from build123d import *

# Parameters (mm, degrees)
BOSS_EXTRUDE4_DEPTH  = 1.5875
M3_CLEARANCE_HOLE3_D = 3
M3_CLEARANCE_HOLE1_D = 3.1
M3_CLEARANCE_HOLE4_D = 2.95
M3_CLEARANCE_HOLE2_D = 3.1
BOSS_EXTRUDE6_DEPTH  = 3.175
FILLET1_R            = 2
FILLET3_R            = 1
FILLET6_R            = 0.5
CUT_EXTRUDE4_DEPTH   = 10
SKETCH29_R           = 1.5
CUT_EXTRUDE5_DEPTH   = 10
SKETCH31_R           = 1.5
CUT_EXTRUDE7_DEPTH   = 10


with BuildPart() as part:
    # Sketch1 → Boss-Extrude4 (new, symmetric)
    with BuildSketch(Plane(origin=(0, 0, 0), x_dir=(1, 0, 0), z_dir=(0, 1, 0))):
        with BuildLine():
            Line((-62.799553621, 32.496136604), (-73.969425011, 32.691107434))
            Line((-73.969425011, 32.691107434), (-77.053684287, 35.88495141))
            ThreePointArc((-77.053684287, 35.88495141), (-84.36642289, 10.358894189), (-83.446216027, -16.178041625))
            Line((-83.446216027, -16.178041625), (-79.680911643, -13.825218315))
            Line((-79.680911643, -13.825218315), (-69.484649137, -16.179210996))
            Line((-69.484649137, -16.179210996), (-43.894490772, -57.132025032))
            Line((-43.894490772, -57.132025032), (-43.894490772, -64.826600275))
            Line((-43.894490772, -64.826600275), (-43.094490772, -64.826600275))
            Line((-43.094490772, -64.826600275), (-34, -64.826600275))
            Line((-34, -64.826600275), (-34, -59.55))
            Line((-34, -59.55), (-34, -58.55))
            Line((-34, -58.55), (-20, -58.55))
            Line((-20, -58.55), (-19.859459165, -59.55))
            Line((-19.859459165, -59.55), (19.859459165, -59.55))
            Line((19.859459165, -59.55), (20, -58.55))
            Line((20, -58.55), (34, -58.55))
            Line((34, -58.55), (34, -59.55))
            Line((34, -59.55), (34, -64.826600275))
            Line((34, -64.826600275), (43.094490772, -64.826600275))
            Line((43.094490772, -64.826600275), (43.894490772, -64.826600275))
            Line((43.894490772, -64.826600275), (43.894490772, -57.132025032))
            Line((43.894490772, -57.132025032), (69.484649137, -16.179210996))
            Line((69.484649137, -16.179210996), (79.680911643, -13.825218315))
            Line((79.680911643, -13.825218315), (83.446216027, -16.178041625))
            ThreePointArc((83.446216027, -16.178041625), (84.610662337, -8.126242604), (85, 0))
            ThreePointArc((85, 0), (82.98964744, 18.377116688), (77.053684287, 35.88495141))
            Line((77.053684287, 35.88495141), (73.969425011, 32.691107434))
            Line((73.969425011, 32.691107434), (62.799553621, 32.496136604))
            Line((62.799553621, 32.496136604), (30.284668021, 63.895396642))
            Line((30.284668021, 63.895396642), (30.089697191, 75.065268032))
            Line((30.089697191, 75.065268032), (33.173956467, 78.259112008))
            ThreePointArc((33.173956467, 78.259112008), (0, 85), (-33.173956467, 78.259112008))
            Line((-33.173956467, 78.259112008), (-30.089697191, 75.065268032))
            Line((-30.089697191, 75.065268032), (-30.284668021, 63.895396642))
            Line((-30.284668021, 63.895396642), (-62.799553621, 32.496136604))
        make_face()
    extrude(amount=BOSS_EXTRUDE4_DEPTH, both=True)

    # M3 Clearance Hole3 (through all)
    with Locations(Plane(origin=(0, -1.5875, 0), x_dir=(-1, 0, 0), z_dir=(0, -1, 0))):
        with Locations((36.5, -50), (36.5, -38), (-36.5, -50), (-36.5, -38)):
            Hole(M3_CLEARANCE_HOLE3_D / 2)

    # M3 Clearance Hole1 (through all)
    with Locations(Plane(origin=(0, 1.5875, 0), x_dir=(1, 0, 0), z_dir=(0, 1, 0))):
        with Locations((-78.542321426, -8.49139241), (78.542321426, -8.49139241), (74.155025063, 27.240269049), (-74.155025063, 27.240269049)):
            Hole(M3_CLEARANCE_HOLE1_D / 2)

    # M3 Clearance Hole4 (through all)
    with Locations(Plane(origin=(0, -1.5875, 0), x_dir=(-1, 0, 0), z_dir=(0, -1, 0))):
        with Locations((-67.099301622, -15.278865202), (-50.141885166, -42.416404279), (-61.062544382, 30.698137949), (-38.043670771, 52.927205804), (50.141885166, -42.416404279), (67.099301622, -15.278865202), (38.043670771, 52.927205804), (61.062544382, 30.698137949)):
            Hole(M3_CLEARANCE_HOLE4_D / 2)

    # M3 Clearance Hole2 (through all)
    with Locations(Plane(origin=(0, 1.5875, 0), x_dir=(1, 0, 0), z_dir=(0, 1, 0))):
        with Locations((27, 76.497766718), (-27, 76.497766718)):
            Hole(M3_CLEARANCE_HOLE2_D / 2)

    # Sketch22 → Boss-Extrude6 (add)
    with BuildSketch(Plane(origin=(0, 1.5875, 0), x_dir=(1, 0, 0), z_dir=(0, 1, 0))):
        Polygon((65.061950694, 32.535626892), (30.245177733, 66.157793715), (30.284668021, 63.895396642), (62.799553621, 32.496136604), align=None)
        Polygon((-30.284668021, 63.895396642), (-30.245177733, 66.157793715), (-65.061950694, 32.535626892), (-62.799553621, 32.496136604), align=None)
        Polygon((43.894490772, -60.151352895), (71.689396914, -15.670204865), (69.484649137, -16.179210996), (43.894490772, -57.132025032), align=None)
        Polygon((-69.484649137, -16.179210996), (-71.689396914, -15.670204865), (-43.894490772, -60.151352895), (-43.894490772, -57.132025032), align=None)
    extrude(amount=-BOSS_EXTRUDE6_DEPTH)

    # Fillet1
    fillet1_edges = [part.edges().sort_by_distance(p)[0] for p in [
        (-30.245177733, 0.79375, -66.157793715),
        (-65.061950694, 0.79375, -32.535626892),
        (-71.689396914, 0.79375, 15.670204865),
        (-43.894490772, 0.79375, 60.151352895),
        (43.894490772, -0.79375, 60.151352895),
        (71.689396914, -0.79375, 15.670204865),
        (65.061950694, 0.79375, -32.535626892),
        (30.245177733, -0.79375, -66.157793715),
        (30.089697191, -0.79375, -75.065268032),
        (73.969425011, -0.79375, -32.691107434),
        (79.680911643, -0.79375, 13.825218315),
        (-79.680911643, -0.79375, 13.825218315),
        (-73.969425011, -0.79375, -32.691107434),
        (-30.089697191, -0.79375, -75.065268032),
    ]]
    fillet(fillet1_edges, radius=FILLET1_R)

    # Fillet3
    fillet3_edges = [part.edges().sort_by_distance(p)[0] for p in [
        (33.173956467, -0.79375, -78.259112008),
        (77.053684287, 0.79375, -35.88495141),
        (83.446216027, -0.79375, 16.178041625),
        (43.894490772, -0.79375, 64.826600275),
        (34, 0.79375, 64.826600275),
        (34, -0.79375, 58.55),
        (-34, -0.79375, 58.55),
        (-34, 0.79375, 64.826600275),
        (-43.894490772, -0.79375, 64.826600275),
        (-83.446216027, -0.79375, 16.178041625),
        (-77.053684287, -0.79375, -35.88495141),
        (-33.173956467, -0.79375, -78.259112008),
    ]]
    fillet(fillet3_edges, radius=FILLET3_R - 0.0001)  # a hair under: the kernel refuses the full size

    # Fillet6
    fillet6_edges = [part.edges().sort_by_distance(p)[0] for p in [
        (20, -0.79375, 58.55),
        (19.859459165, -0.79375, 59.55),
        (-19.859459165, 0.79375, 59.55),
        (-20, 0.79375, 58.55),
    ]]
    fillet(fillet6_edges, radius=FILLET6_R)

    # Sketch28 → Cut-Extrude4 (cut)
    with BuildSketch(Plane(origin=(0, 1.5875, 0), x_dir=(1, 0, 0), z_dir=(0, 1, 0))):
        with BuildLine():
            Line((-26.25, -9.55), (-26.25, -59.55))
            Line((-26.25, -59.55), (26.25, -59.55))
            Line((26.25, -59.55), (26.25, -9.55))
            Line((26.25, -9.55), (21.2, -9.55))
            Line((21.2, -9.55), (21.2, -1.5))
            Line((21.2, -1.5), (4.195235393, -1.5))
            ThreePointArc((4.195235393, -1.5), (0, 2.5), (-4.195235393, -1.5))
            Line((-4.195235393, -1.5), (-21.2, -1.5))
            Line((-21.2, -1.5), (-21.2, -9.55))
            Line((-21.2, -9.55), (-26.25, -9.55))
        make_face()
    extrude(amount=-CUT_EXTRUDE4_DEPTH, mode=Mode.SUBTRACT)

    # Sketch29 → Cut-Extrude5 (cut)
    with BuildSketch(Plane(origin=(0, 1.5875, 0), x_dir=(1, 0, 0), z_dir=(0, 1, 0))):
        with Locations(Location((30.25, -53.55, 0), (0, 0, 270))):
            Circle(SKETCH29_R)
        with Locations(Location((-30.25, -53.55, 0), (0, 0, 270))):
            Circle(SKETCH29_R)
    extrude(amount=-CUT_EXTRUDE5_DEPTH, mode=Mode.SUBTRACT)

    # Sketch31 → Cut-Extrude7 (cut)
    with BuildSketch(Plane(origin=(0, 1.5875, 0), x_dir=(1, 0, 0), z_dir=(0, 1, 0))):
        with Locations(Location((-26, -6.55, 0), (0, 0, 270))):
            Circle(SKETCH31_R)
        with Locations(Location((26, -6.55, 0), (0, 0, 270))):
            Circle(SKETCH31_R)
        with Locations(Location((-26, 19.8, 0), (0, 0, 270))):
            Circle(SKETCH31_R)
        with Locations(Location((26, 19.8, 0), (0, 0, 270))):
            Circle(SKETCH31_R)
    extrude(amount=-CUT_EXTRUDE7_DEPTH, mode=Mode.SUBTRACT)


solid = part.part
Can you work these out from the model? Positions are in its coordinate system, mm. Give positions to 0.01 mm unless a question says otherwise; leave off trailing zeros. Loops run counter-clockwise (first coordinate to the right, second up) from the corner with the lowest first, then second, coordinate; pieces in that order, holes last. Notation, with made-up numbers: (85, 75.5) - (100, 75.5) arc R24 cw to (100, 113.5) - close; hole circle Ø1 at (44.5, 61). An arc over 180 degrees is marked (long way). Return JSON: item names as keys, results as strings.
1. I'm going to push flat-ended pins straight in: pin 1 Ø0.9 at (y, z) = (0, 63) entering from +X; pin 2 Ø1 at (x, y) = (12, -0.5) entering from +Z; pin 3 Ø1.5 at (y, z) = (0.5, -20) entering from -X; pin 4 Ø2.5 at (x, z) = (61.06, -30.7) entering from +Y. Where does each tip first touch, or does it pass through?
Output values:
{"pin 1": "stops at x = 43.89", "pin 2": "stops at z = 1.5", "pin 3": "stops at x = -82.79", "pin 4": "passes through"}
2. I want a section at C-C on y = -0.85. Give the number of separate pieces and of enclosed holes in the cut face, and give its area (3 significant figures).
Output values:
{"separate pieces": "1", "enclosed holes": "24", "area": "14,300 mm²"}
3. I want a section at A-A on z = 19. Please give me the cut outline in (x, y), and give its area (3 significant figures).
Output values:
{"outline": "(-69.61, -1.59) - (-26.25, -1.59) - (-26.25, 1.59) - (-69.61, 1.59) - close; (26.25, -1.59) - (69.61, -1.59) - (69.61, 1.59) - (26.25, 1.59) - close", "area": "275 mm²"}
4. We'd pull the mould along X, two halves only. Please class faces 1 (the face through (-84.323, 0.022, -10.709)), 2 (the face through (0.1, 0, -2.5)), 3 (the face through (0, 0, -85)): +X half, -X half, draft (parallel to the pull), parting line (faces both ways), or undercut.
Output values:
{"face 1": "-X half", "face 2": "undercut", "face 3": "parting line"}
5. If I drill on line 1 (X direction, y = 0.45, z = 6.55); line 2 (Z direction, x = -36.5, y = -0.4); line 3 (Z direction, x = 25, y = -1.35), over which ranges is the centre line in solid material (lowest first)?
Output values:
{"line 1": "x = -84.75 to -27.5, -24.5 to -21.2, 21.2 to 24.5, 27.5 to 84.75", "line 2": "z = -60.12 to 36.5, 39.5 to 48.5, 51.5 to 64.83", "line 3": "z = -81.24 to -20.92, -18.68 to 5.43, 7.67 to 9.55"}
6. I want a section at B-B on x = 0. Please give me the cut outline in (y, z).
Output values:
{"outline": "(-1.59, -85) - (1.59, -85) - (1.59, -2.5) - (-1.59, -2.5) - close"}
